```python
from build123d import *

# Parameters (mm, degrees)
F0_R          = 25.4
F1_DEPTH      = 863.6
F2_R          = 25.4
F3_DEPTH      = 50.8
F3_DEPTH_BACK = 76.2
F3_TAPER_BACK = 10
F4_R          = 38.1
F5_DEPTH      = 762
F5_DEPTH_BACK = 508


with BuildPart() as f1:
    # F0 (on Top) → F1 (new body)
    with BuildSketch(Plane.XY):
        with Locations((0, 50.8)):
            Circle(F0_R)
    extrude(amount=F1_DEPTH)



with BuildPart() as f1b:
    # F0 (on Top) → F1, piece 2 (new body)
    with BuildSketch(Plane.XY):
        with Locations((-43.9940905122, -25.4)):
            Circle(F0_R)
    extrude(amount=F1_DEPTH)


with BuildPart() as f1c:
    # F0 (on Top) → F1, piece 3 (new body)
    with BuildSketch(Plane.XY):
        with Locations((43.9940905122, -25.4)):
            Circle(F0_R)
    extrude(amount=F1_DEPTH)


with BuildPart() as f1_1:
    add(f1.part)

    add(f1b.part)  # F3 merges F1b

    add(f1c.part)  # F3 merges F1c
    # F2 (on face) → F3 (join, two sides)
    with BuildSketch(Plane.XY.offset(863.6)) as f3_sk:
        Polygon((59.9760856868, 82.55), (-59.9760856868, 82.55), (-97.0433451535, -31.5312942287), (0, -102.0374115426), (97.0433451535, -31.5312942287), align=None)
        with Locations((-43.9940905122, -25.4)):
            Circle(F2_R, mode=Mode.SUBTRACT)
        with Locations((-43.9940905122, -25.4)):
            Circle(F2_R)
    extrude(amount=-F3_DEPTH)
    extrude(f3_sk.sketch, amount=F3_DEPTH_BACK, taper=F3_TAPER_BACK)

    # F4 (on face) → F5 (join, two sides)
    with BuildSketch(Plane.XY.offset(939.8)) as f5_sk:
        Circle(F4_R)
    extrude(amount=F5_DEPTH)
    extrude(f5_sk.sketch, amount=-F5_DEPTH_BACK)


solid = f1_1.part
```
Could you check a few things on this model? Use its own coordinates, in mm. A direction names the side the tool comes from. Round coordinates to 2 decimals unless told otherwise and drop trailing zeros. Loops run counter-clockwise (first coordinate to the right, second up) from the corner with the lowest first, then second, coordinate; pieces in that order, holes last.
Q1. I want a section at C-C (z = 693.5). Write out the boundary of the cut face in (x, y), and give its area (3 significant figures).
Q2. On a 3-axis mill with a long thin cutter (end or side, diameter ignored), from which of +Z, -Z, +X, -X, +Y, -Y can I reach the whole of each face in a straight line? I mean faces 5 (the cylindrical face through (-30.235, -23.183, 1315.466)), 6 (the flat face through (20, 33, 812.8)), 7 (the flat face through (-44, -25, 0)). Say none if no direction works.
Q3. I want a section at A-A (y = -69). Write out the boundary of the cut face in (x, z).
Q4. I want a section at B-B (z = 1348.5). Write out the boundary of the cut face in (x, y), and give its area (3 significant figures).
Q5. Please list where these lines run through material, in increasing order: L1, parallel to Z at x = 16, y = 44; L2, parallel to X at y = -25, z = 374.5; L3, parallel to Z at x = 3, y = -67.5.
Q6. Thinking about a two-plate mould opening in X: for faces 1 (the flat face through (45.31, -60.93, 901.17)), 2 (the flat face through (-78.25, 26.31, 838.56)), 3 (the flat face through (1, 82.55, 839)), 4 (the cylindrical face through (67.457, -35.128, 400.71)), which applies, pulls with the +X half, pulls with the -X half, needs draft (parallel to the pull), parting line crosses it, or undercut?
Q7. For P1, Ø3, axis at x = 21, y = 46.5, coming from the -Z side; P2, Ø5, axis at y = -1, z = 989.5, coming from the -X side; P3, Ø1, axis at y = -27.5, z = 484.5, coming from the -X side; P4, Ø4, axis at x = -9.5, z = 289.5, coming from the +Y side, each with a flat end and sliding along its axis, tell me the tip position at first contact or that it passes through.
Answer below:
1. outline: (-38.09, -0.69) arc R25.4 ccw (long way) to (-19.65, -32.64) arc R38.1 ccw to (19.65, -32.64) arc R25.4 ccw (long way) to (38.09, -0.69) arc R38.1 ccw to (18.45, 33.34) arc R25.4 ccw (long way) to (-18.45, 33.34) arc R38.1 ccw to start
1. area: 9,680 mm2
2. face 5: +Z
2. face 6: -Z
2. face 7: -Z, +X, -X, +Y, -Y
3. outline: (-45.47, 812.8) - (45.47, 812.8) - (45.47, 863.6) - (22.61, 939.8) - (-22.61, 939.8) - (-45.47, 863.6) - close
4. outline: circle Ø76.2 at (0, 0)
4. area: 4,560 mm2
5. L1: z = 0 to 939.8
5. L2: x = -69.39 to -18.6, 18.6 to 69.39
5. L3: z = 812.8 to 939.8
6. face 1: pulls with the +X half
6. face 2: pulls with the -X half
6. face 3: needs draft
6. face 4: undercut
7. P1: stops at z = 0
7. P2: stops at x = -38.1
7. P3: stops at x = -69.34
7. P4: stops at y = 75.07
